Verification items for the finished model (mm, model axes). Face numbers are marked on the shaded views. A direction names the side the tool comes from. Coordinates: 2 decimals unless noted, no trailing zeros. Order: outer loops, then holes, each group sorted by start corner. A loop starts at its lowest first (then second) coordinate and runs counter-clockwise, first axis right, second up. Notation, with made-up numbers: (-20.75, 61.25) -> (11.25, 61.25) arc R15 ccw to (11.25, 85.25) -> close; hole circle Ø4 at (56.25, -33.75). An arc over 180 degrees is marked (long way). Write item = value, one per line. Start each with the question number.
1. Set-up check for the marked faces 1, 2 and 3: record each of +Z, -Z, +X, -X, +Y, -Y from which the full face is reachable in a straight line by a thin tool's end or side.
2. Go/stop test with flat-tipped pins: P1, Ø12, axis at x = -44.5, y = -16, coming from the +Z side; P2, Ø6, axis at x = -35.5, y = -40.5, coming from the +Z side; P3, Ø7, axis at x = -12.59, y = -44.41, coming from the -Z side; P4, Ø12, axis at x = -11.5, z = 18.5, coming from the +Y side. Record where each tip stops, or that it passes through.
3. Cross-section at A-A on x = -28.5. Record the cut outline in (y, z).
4. Thickness scan on line 1 along Y through (x, z) = (-37, 30); line 2 along Z through (x, y) = (-50, -30.5); line 3 along Y through (x, z) = (-51, 27). Record the ranges inside material, lowest first. Write a range as from..to.
5. Cross-section at C-C on x = -20. Record the cut outline in (y, z), plus the area to 3 significant figures.
6. Cross-section at B-B on z = -17.5. Record the cut outline in (x, y).
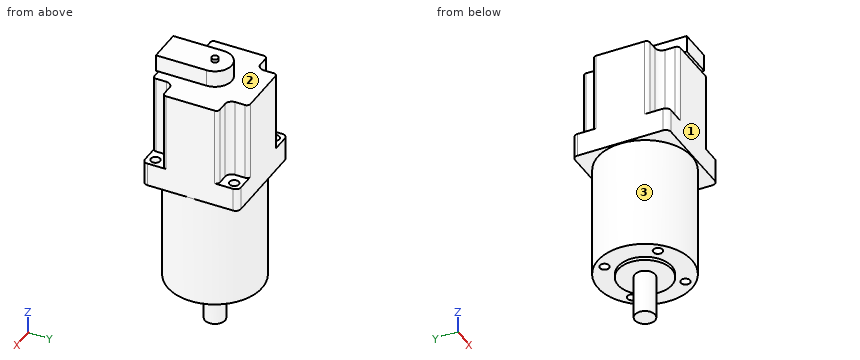
from build123d import *

# Parameters (mm, degrees)
BOSS_EXTRUDE1_DEPTH            = 56
SKETCH2_W                      = 19.654725719
SKETCH2_H                      = 18.883952161
CUT_EXTRUDE1_DEPTH             = 47
FILLET1_R                      = 2
FILLET2_R                      = 4
M5_CLEARANCE_HOLE2_D           = 5.5
M5_CLEARANCE_HOLE2_CSINK_D     = 5.55
M5_CLEARANCE_HOLE2_CSINK_ANGLE = 90
SKETCH6_R                      = 1.95
BOSS_EXTRUDE2_DEPTH            = 12
BOSS_EXTRUDE3_DEPTH            = 5
SKETCH8_R                      = 28
BOSS_EXTRUDE4_DEPTH            = 67
SKETCH9_R                      = 16
BOSS_EXTRUDE5_DEPTH            = 2
CIRPATTERN1_COUNT              = 4
SKETCH14_R                     = 6
BOSS_EXTRUDE6_DEPTH            = 26
SKETCH17_R                     = 1.907386748
BOSS_EXTRUDE7_DEPTH            = 10


with BuildPart() as part:
    # Sketch1 → Boss-Extrude1 (new body)
    with BuildSketch(Plane.XY):
        with BuildLine():
            Line((-3, 0), (-54, 0))
            ThreePointArc((-54, 0), (-56.121320344, -0.878679656), (-57, -3))
            Line((-57, -3), (-57, -54))
            ThreePointArc((-57, -54), (-56.121320344, -56.121320344), (-54, -57))
            Line((-54, -57), (-3, -57))
            ThreePointArc((-3, -57), (-0.878679656, -56.121320344), (0, -54))
            Line((0, -54), (0, -3))
            ThreePointArc((0, -3), (-0.878679656, -0.878679656), (-3, 0))
        make_face()
    extrude(amount=BOSS_EXTRUDE1_DEPTH)

    # Sketch2 → Cut-Extrude1 (cut)
    with BuildSketch(Plane.XY.offset(56)):
        with Locations((-54.827362859, -2.558023919)):
            Rectangle(SKETCH2_W, SKETCH2_H)
        with Locations((-2.17263714, -2.558023919)):
            Rectangle(SKETCH2_W, SKETCH2_H)
        with Locations((-2.17263714, -54.44197608)):
            Rectangle(SKETCH2_W, SKETCH2_H)
        with Locations((-54.827362859, -54.44197608)):
            Rectangle(SKETCH2_W, SKETCH2_H)
    extrude(amount=-CUT_EXTRUDE1_DEPTH, mode=Mode.SUBTRACT)

    # Fillet1
    fillet1_edges = [part.edges().sort_by_distance(p)[0] for p in [
        (-57, -45, 32.5),
        (-45, -57, 32.5),
        (-12, -57, 32.5),
        (0, -45, 32.5),
        (0, -12, 32.5),
        (-12, 0, 32.5),
        (-45, 0, 32.5),
        (-57, -12, 32.5),
    ]]
    fillet(fillet1_edges, radius=FILLET1_R)

    # Fillet2
    fillet2_edges = [part.edges().sort_by_distance(p)[0] for p in [
        (-45, -45, 32.5),
        (-12, -45, 32.5),
        (-12, -12, 32.5),
        (-45, -12, 32.5),
    ]]
    fillet(fillet2_edges, radius=FILLET2_R)

    # M5 Clearance Hole2 (through all)
    with Locations(Plane(origin=(0, 0, 0), x_dir=(-1, 0, 0), z_dir=(0, 0, -1))):
        with Locations((51.921563773, -4.957706516), (4.997949753, -4.957706516), (4.997949753, -51.800834063), (51.921563773, -52.283752904)):
            CounterSinkHole(M5_CLEARANCE_HOLE2_D / 2, M5_CLEARANCE_HOLE2_CSINK_D / 2, counter_sink_angle=M5_CLEARANCE_HOLE2_CSINK_ANGLE)

    # Sketch6 → Boss-Extrude2 (add)
    with BuildSketch(Plane.XY.offset(56)):
        with Locations((-28.5, -28.5)):
            Circle(SKETCH6_R)
    extrude(amount=BOSS_EXTRUDE2_DEPTH)

    # Sketch7 → Boss-Extrude3 (add)
    with BuildSketch(Plane(origin=(0, 0, 0), x_dir=(-1, 0, 0), z_dir=(0, 0, -1))):
        with BuildLine():
            Line((57, -54), (57, -3))
            ThreePointArc((57, -3), (56.121320344, -0.878679656), (54, 0))
            Line((54, 0), (3, 0))
            ThreePointArc((3, 0), (0.878679656, -0.878679656), (0, -3))
            Line((0, -3), (0, -54))
            ThreePointArc((0, -54), (0.878679656, -56.121320344), (3, -57))
            Line((3, -57), (54, -57))
            ThreePointArc((54, -57), (56.121320344, -56.121320344), (57, -54))
        make_face()
    extrude(amount=BOSS_EXTRUDE3_DEPTH)

    # Sketch8 → Boss-Extrude4 (add)
    with BuildSketch(Plane(origin=(0, 0, -5), x_dir=(-1, 0, 0), z_dir=(0, 0, -1))):
        with Locations((28.5, -28.5)):
            Circle(SKETCH8_R)
    extrude(amount=BOSS_EXTRUDE4_DEPTH)

    # Sketch9 → Boss-Extrude5 (add)
    with BuildSketch(Plane(origin=(0, 0, -72), x_dir=(-1, 0, 0), z_dir=(0, 0, -1))):
        with Locations((28.5, -28.5)):
            Circle(SKETCH9_R)
    extrude(amount=BOSS_EXTRUDE5_DEPTH)

    # Sketch13 → M5 Clearance Hole1 (revolve, cut)
    with BuildSketch(Plane(origin=(-44.409902577, -12.590097423, -72), x_dir=(0, 1, 0), z_dir=(1, 0, 0))):
        Polygon((0, 0), (0, 21.652366702), (2.75, 20), (2.75, 0.025), (2.775, 0), align=None)
    m5_clearance_hole1 = revolve(axis=Axis((-44.409902577, -12.590097423, -78.35), (0, 0, 1)), mode=Mode.SUBTRACT)

    # CirPattern1: M5 Clearance Hole1 ×4 about axis
    cirpattern1_axis = Axis((-28.5, -28.5, 0), (0, 0, 1))
    for i in range(1, CIRPATTERN1_COUNT):
        add(m5_clearance_hole1.rotate(cirpattern1_axis, i * 360 / CIRPATTERN1_COUNT), mode=Mode.SUBTRACT)

    # Sketch14 → Boss-Extrude6 (add)
    with BuildSketch(Plane(origin=(0, 0, -74), x_dir=(-1, 0, 0), z_dir=(0, 0, -1))):
        with Locations((28.5, -28.5)):
            Circle(SKETCH14_R)
    extrude(amount=BOSS_EXTRUDE6_DEPTH)

    # Sketch17 → Boss-Extrude7 (add)
    with BuildSketch(Plane.XY.offset(56)):
        with BuildLine():
            Line((-18.5, -28.5), (-18.5, -58.5))
            Line((-18.5, -58.5), (-38.5, -58.5))
            Line((-38.5, -58.5), (-38.5, -28.5))
            ThreePointArc((-38.5, -28.5), (-28.5, -18.5), (-18.5, -28.5))
        make_face()
        with Locations((-28.5, -28.5)):
            Circle(SKETCH17_R, mode=Mode.SUBTRACT)
    extrude(amount=BOSS_EXTRUDE7_DEPTH)


solid = part.part
Worked out:
q1.face_1 = -Z, +X, -X, -Y
q1.face_2 = +Z, +Y
q1.face_3 = -Z
q2.P1 = 56
q2.P2 = 66
q2.P3 = -72
q2.P4 = 0
q3.outline = (-58.5, 56) -> (-57, 56) -> (-57, -5) -> (-56.5, -5) -> (-56.5, -72) -> (-44.5, -72) -> (-44.5, -74) -> (-34.5, -74) -> (-34.5, -100) -> (-22.5, -100) -> (-22.5, -74) -> (-12.5, -74) -> (-12.5, -72) -> (-0.5, -72) -> (-0.5, -5) -> (0, -5) -> (0, 56) -> (-18.5, 56) -> (-18.5, 66) -> (-26.55, 66) -> (-26.55, 68) -> (-30.45, 68) -> (-30.45, 66) -> (-58.5, 66) -> close
q4.line_1 = -57..0
q4.line_2 = -72..56
q4.line_3 = -45..-12
q5.outline = (-58.5, 56) -> (-57, 56) -> (-57, -5) -> (-55.18, -5) -> (-55.18, -72) -> (-42.06, -72) -> (-42.06, -74) -> (-14.94, -74) -> (-14.94, -72) -> (-1.82, -72) -> (-1.82, -5) -> (0, -5) -> (0, 56) -> (-23.23, 56) -> (-23.23, 66) -> (-58.5, 66) -> close
q5.area = 7,460 mm²
q6.outline = circle Ø56 at (-28.5, -28.5)
